from build123d import *

# Parameters (mm, degrees)
BOSS_EXTRUDE1_DEPTH     = 22
BOSS_EXTRUDE2_DEPTH     = 64
SKETCH3_R               = 3
CUT_EXTRUDE1_DEPTH      = 65
SKETCH4_R               = 6
CUT_EXTRUDE2_DEPTH      = 52
M4_TAPPED_HOLE1_D       = 3.3
M4_TAPPED_HOLE1_DEPTH   = 14
M4_TAPPED_HOLE1_TIP     = 0.991420021
CUT_EXTRUDE3_REACH      = 93.679
CUT_EXTRUDE3_END_RADIUS = 3
SKETCH8_R               = 2.5
SKETCH8_R_2             = 1.5
SKETCH9_R               = 1
CUT_EXTRUDE4_DEPTH      = 15
CHAMFER1_SIZE           = 1


with BuildPart() as part:
    # Sketch1 → Boss-Extrude1 (new body)
    with BuildSketch(Plane(origin=(0, 0, 0), x_dir=(1, 0, 0), z_dir=(0, 1, 0))):
        with BuildLine():
            Line((-3.31662479, -5), (3.31662479, -5))
            ThreePointArc((3.31662479, -5), (0, 6), (-3.31662479, -5))
        make_face()
    extrude(amount=BOSS_EXTRUDE1_DEPTH)

    # Sketch2 → Boss-Extrude2 (add)
    with BuildSketch(Plane(origin=(0, 22, 0), x_dir=(1, 0, 0), z_dir=(0, 1, 0))):
        with BuildLine():
            Line((-13, 7.483314774), (-13, -7.483314774))
            ThreePointArc((-13, -7.483314774), (15, 0), (-13, 7.483314774))
        make_face()
    extrude(amount=BOSS_EXTRUDE2_DEPTH)

    # Sketch3 → Cut-Extrude1 (cut)
    with BuildSketch(Plane(origin=(0, 86, 0), x_dir=(1, 0, 0), z_dir=(0, 1, 0))):
        with Locations(Location((-8, 0, 0), (0, 0, 270))):
            Circle(SKETCH3_R)
    extrude(amount=-CUT_EXTRUDE1_DEPTH, mode=Mode.SUBTRACT)

    # Sketch4 → Cut-Extrude2 (cut)
    with BuildSketch(Plane(origin=(0, 86, 0), x_dir=(1, 0, 0), z_dir=(0, 1, 0))):
        with Locations(Location((5, 0, 0), (0, 0, 270))):
            Circle(SKETCH4_R)
    extrude(amount=-CUT_EXTRUDE2_DEPTH, mode=Mode.SUBTRACT)

    # M4 Tapped Hole1
    with Locations(Plane(origin=(0, 86, 0), x_dir=(1, 0, 0), z_dir=(0, 1, 0))):
        with Locations((0, 9), (0, -9)):
            Hole(M4_TAPPED_HOLE1_D / 2, depth=M4_TAPPED_HOLE1_DEPTH)
            with Locations((0, 0, -(M4_TAPPED_HOLE1_DEPTH + M4_TAPPED_HOLE1_TIP / 2))):  # 118° drill point
                Cone(0, M4_TAPPED_HOLE1_D / 2, M4_TAPPED_HOLE1_TIP, mode=Mode.SUBTRACT)

    # Cut-Extrude3: up to this cylinder (the profile starts outside it)
    cut_extrude3_end = Plane(origin=(-8, 39.5, 0), z_dir=(0, 1, 0)) * Cylinder(CUT_EXTRUDE3_END_RADIUS, 223.358, mode=Mode.PRIVATE)
    # Sketch8 → Cut-Extrude3 (cut, up to the surface)
    with BuildSketch(Plane.ZY.offset(13), mode=Mode.PRIVATE) as cut_extrude3_sk1:
        with Locations((0, 54)):
            Circle(SKETCH8_R)
    cut_extrude3_tool1 = extrude(cut_extrude3_sk1.sketch, amount=-CUT_EXTRUDE3_REACH, mode=Mode.PRIVATE) - cut_extrude3_end
    add(cut_extrude3_tool1.solids().sort_by_distance((-13, 54, 0))[0], mode=Mode.SUBTRACT)
    # Sketch8 → Cut-Extrude3 (cut, up to the surface)
    with BuildSketch(Plane.ZY.offset(13), mode=Mode.PRIVATE) as cut_extrude3_sk2:
        with Locations((0, 25)):
            Circle(SKETCH8_R_2)
    cut_extrude3_tool2 = extrude(cut_extrude3_sk2.sketch, amount=-CUT_EXTRUDE3_REACH, mode=Mode.PRIVATE) - cut_extrude3_end
    add(cut_extrude3_tool2.solids().sort_by_distance((-13, 25, 0))[0], mode=Mode.SUBTRACT)

    # Sketch9 → Cut-Extrude4 (cut)
    with BuildSketch(Plane.ZY.offset(13)):
        with Locations((0, 76)):
            Circle(SKETCH9_R)
        with Locations((0, 34)):
            Circle(SKETCH9_R)
    extrude(amount=-CUT_EXTRUDE4_DEPTH, mode=Mode.SUBTRACT)

    # Chamfer1
    chamfer1_edges = [part.edges().sort_by_distance(p)[0] for p in [
        (0, 0, 5),
        (0, 0, -6),
    ]]
    chamfer(chamfer1_edges, length=CHAMFER1_SIZE - 0.0001)  # a hair under: the kernel refuses the full size


solid = part.part
Input: part model. Units: mm. Frame: model coordinates. A direction names the side the tool comes from. Give positions to 0.01 mm unless a question says otherwise; leave off trailing zeros. Loops run counter-clockwise (first coordinate to the right, second up) from the corner with the lowest first, then second, coordinate; pieces in that order, holes last. Notation, with made-up numbers: (-13.75, 20.25) -> (14.25, 20.25) arc R24 cw to (14.25, 48.25) -> close; hole circle Ø11 at (34, -15). An arc over 180 degrees is marked (long way). Answer as a JSON object with one key per item and string values. Group by question number.
Item 1: Cut plane B-B, the plane z = 0. State how many separate pieces and enclosed holes the cut face has, and give its area (3 significant figures).
Item 2: Cut plane D-D, the plane y = 25. Return the cut outline in (x, z).
Item 3: Cut plane C-C, the plane x = -8. Return the cut outline in (y, z).
Item 4: Reachability of faces 1 (the flat face through (0, 11, 5)), 2 (the cylindrical face through (6.802, 60.364, 5.723)), 3 (the cylindrical face through (-3, 75, 0)) from +Z, -Z, +X, -X, +Y, -Y: full face, straight path, thin tool, end or side. Return the list, or none.
Item 5: Line query: probe 1 along Y at (x, z) = (-4.2, 0); probe 2 along Y at (x, z) = (-12.3, 0); probe 3 along X at (y, z) = (52.5, 0). Output: solid intervals per line, ascending.
Item 6: Pull-direction query (X, two-part tool) for faces 4 (the flat face through (-13, 54, -3)), 5 (the cylindrical face through (0, 11, -6)), 6 (the flat face through (7, 22, 0)), 7 (the conical face through (-0.04, 71.18, 8.72)); classes: released by +X, released by -X, zero draft, split by the parting line, or undercut.
Item 7: Pin query (flat end, axial travel): P1, Ø1.8, axis at y = 76, z = 0, coming from the -X side; P2, Ø4.5, axis at x = 0, z = -9, coming from the -Y side; P3, Ø1.8, axis at y = 34, z = 0, coming from the -X side. Return the tip coordinate at first contact, or that it passes through.
Item 8: Cut plane A-A, the plane y = 76. Return the cut outline in (x, z), and give its area (3 significant figures).
Checks:
{
 "1": {"separate pieces": "8", "enclosed holes": "0", "area": "1,000 mm²"},
 "2": {"outline": "(-13, -7.48) arc R15 ccw (long way) to (-13, 7.48) -> (-13, 1.5) -> (-10.6, 1.5) arc R3 cw (long way) to (-10.6, -1.5) -> (-13, -1.5) -> close"},
 "3": {"outline": "(22, -12.69) -> (86, -12.69) -> (86, -3) -> (22, -3) -> close; (22, 3) -> (86, 3) -> (86, 12.69) -> (22, 12.69) -> close"},
 "4": {"face 1": "+Z, +X, -X, -Y", "face 2": "+Y", "face 3": "-X"},
 "5": {"probe 1": "y = 0 to 33, 35 to 75, 77 to 86", "probe 2": "y = 22 to 23.5, 26.5 to 33, 35 to 51.5, 56.5 to 75, 77 to 86", "probe 3": "x = -5 to -1, 11 to 15"},
 "6": {"face 4": "released by -X", "face 5": "split by the parting line", "face 6": "zero draft", "face 7": "undercut"},
 "7": {"P1": "stops at x = 10.93", "P2": "stops at y = 22", "P3": "stops at x = 2"},
 "8": {"outline": "(-13, -7.48) arc R15 ccw (long way) to (-13, 7.48) -> (-13, 1) -> (-10.83, 1) arc R3 cw to (-5.17, 1) -> (-0.92, 1) arc R6 cw (long way) to (-0.92, -1) -> (-5.17, -1) arc R3 cw to (-10.83, -1) -> (-13, -1) -> close; hole circle Ø3.3 at (0, -9); hole circle Ø3.3 at (0, 9)", "area": "516 mm²"}
}
